from build123d import *

# Parameters (mm, degrees)
BOSS_EXTRUDE1_DEPTH     = 1.5
BOSS_EXTRUDE2_DEPTH     = 280
SKETCH4_W               = 410
SKETCH4_H               = 42.385541564
BOSS_EXTRUDE3_DEPTH     = 30
CUT_EXTRUDE1_DEPTH      = 616.233320702
CUT_EXTRUDE1_DEPTH_BACK = 616.233320702
SKETCH8_R               = 4.39
SKETCH8_R_2             = 2.39
BOSS_EXTRUDE5_DEPTH     = 15
SKETCH10_R              = 3
CUT_EXTRUDE2_DEPTH      = 1.5
SKETCH15_W              = 15
SKETCH15_H              = 1.5
SKETCH15_W_2            = 20
BOSS_EXTRUDE6_DEPTH     = 13
BOSS_EXTRUDE7_DEPTH     = 1.5
BOSS_EXTRUDE8_DEPTH     = 1.5
SKETCH20_R              = 2.415919743
SKETCH20_R_2            = 2
CUT_EXTRUDE5_DEPTH      = 1.5
SKETCH5_R               = 2
SKETCH5_R_2             = 10
CUT_EXTRUDE7_DEPTH      = 1.5
SKETCH21_W              = 300
SKETCH21_H              = 1.5
BOSS_EXTRUDE9_DEPTH     = 10
SKETCH22_W              = 300
SKETCH22_H              = 1.5
BOSS_EXTRUDE10_DEPTH    = 10
BOSS_EXTRUDE11_DEPTH    = 0.75
BOSS_EXTRUDE12_DEPTH    = 0.75
BOSS_EXTRUDE13_DEPTH    = 0.75
BOSS_EXTRUDE14_DEPTH    = 0.75
SKETCH27_W              = 200
SKETCH27_H              = 1.5
BOSS_EXTRUDE15_DEPTH    = 10
BOSS_EXTRUDE16_DEPTH    = 0.75
BOSS_EXTRUDE17_DEPTH    = 0.75
SKETCH30_R              = 24
SKETCH30_R_2            = 1.5
CUT_EXTRUDE8_DEPTH      = 1.5
SKETCH33_R              = 2
CUT_EXTRUDE9_DEPTH      = 1.5


with BuildPart() as part:
    # Sketch1 → Boss-Extrude1 (new body)
    with BuildSketch(Plane(origin=(0, 0, 0), x_dir=(1, 0, 0), z_dir=(0, 1, 0))):
        Polygon((-205, 237.826300096), (205, 237.826300096), (205, -292.173699904), (155, -292.173699904), (155, -362.173699904), (-205, -362.173699904), align=None)
    extrude(amount=BOSS_EXTRUDE1_DEPTH)

    # Sketch2 → Boss-Extrude2 (add)
    with BuildSketch(Plane(origin=(0, 1.5, 0), x_dir=(1, 0, 0), z_dir=(0, 1, 0))):
        Polygon((-205, 237.826300096), (-205, -362.173699904), (155, -362.173699904), (155, -292.173699904), (205, -292.173699904), (205, 237.826300096), align=None)
        Polygon((-203.5, 236.326300096), (-203.5, -360.673699904), (153.5, -360.673699904), (153.5, -290.673699904), (203.5, -290.673699904), (203.5, 236.326300096), align=None, mode=Mode.SUBTRACT)
    extrude(amount=BOSS_EXTRUDE2_DEPTH)

    # Sketch4 → Boss-Extrude3 (add)
    with BuildSketch(Plane(origin=(0, 0, -237.826300096), x_dir=(-1, 0, 0), z_dir=(0, 0, -1))):
        with Locations((0, 213.483316708)):
            Rectangle(SKETCH4_W, SKETCH4_H)
    extrude(amount=BOSS_EXTRUDE3_DEPTH)

    # Sketch3 → Cut-Extrude1 (cut, two sides: drawn at the far end of the back side and taken through both)
    with BuildSketch(Plane.ZY.offset(205).offset(-CUT_EXTRUDE1_DEPTH_BACK)):
        Polygon((362.173699904, 121.117558148), (228.195222706, 281.5), (362.173699904, 281.5), align=None)
    extrude(amount=CUT_EXTRUDE1_DEPTH + CUT_EXTRUDE1_DEPTH_BACK, mode=Mode.SUBTRACT)

    # Sketch8 → Boss-Extrude5 (add)
    # profile 1 of 2: a face of its own
    with BuildSketch(Plane(origin=(-203.5, 0, 0), x_dir=(0, 0, -1), z_dir=(1, 0, 0))):
        with Locations((-265.673699904, 172.2)):
            Circle(SKETCH8_R)
        with Locations((-265.673699904, 172.2)):
            Circle(SKETCH8_R_2, mode=Mode.SUBTRACT)
    # profile 2 of 2: a face of its own
    with BuildSketch(Plane(origin=(-203.5, 0, 0), x_dir=(0, 0, -1), z_dir=(1, 0, 0))):
        with Locations((-265.673699904, 16.5)):
            Circle(SKETCH8_R)
        with Locations((-265.673699904, 16.5)):
            Circle(SKETCH8_R_2, mode=Mode.SUBTRACT)
    extrude(amount=BOSS_EXTRUDE5_DEPTH)

    # Sketch10 → Cut-Extrude2 (cut)
    with BuildSketch(Plane.ZY.offset(-153.5)):
        with BuildLine():
            Line((334.423699904, 90.5), (320.423699904, 90.5))
            Line((320.423699904, 90.5), (320.423699904, 87.5))
            Line((320.423699904, 87.5), (316.173699904, 87.5))
            ThreePointArc((316.173699904, 87.5), (305.173699904, 76.5), (316.173699904, 65.5))
            Line((316.173699904, 65.5), (338.673699904, 65.5))
            ThreePointArc((338.673699904, 65.5), (349.673699904, 76.5), (338.673699904, 87.5))
            Line((338.673699904, 87.5), (334.423699904, 87.5))
            Line((334.423699904, 87.5), (334.423699904, 90.5))
        make_face()
        with Locations((301.473699904, 103.45)):
            Circle(SKETCH10_R)
        with Locations((353.373699904, 103.45)):
            Circle(SKETCH10_R)
        with Locations((301.473699904, 49.55)):
            Circle(SKETCH10_R)
        with Locations((353.373699904, 49.55)):
            Circle(SKETCH10_R)
    extrude(amount=-CUT_EXTRUDE2_DEPTH, mode=Mode.SUBTRACT)

    # Sketch15 → Boss-Extrude6 (add)
    with BuildSketch(Plane.ZY.offset(-203.5)):
        with Locations((-143.826300096, 251.386283415)):
            Rectangle(SKETCH15_W, SKETCH15_H)
        with Locations((136.673699904, 251.386283415)):
            Rectangle(SKETCH15_W_2, SKETCH15_H)
    extrude(amount=BOSS_EXTRUDE6_DEPTH)

    # Sketch17 → Boss-Extrude7 (add)
    with BuildSketch(Plane.XY.offset(-136.326300096)):
        Polygon((203.5, 250.636283415), (203.5, 235.636283415), (190.5, 250.636283415), align=None)
    extrude(amount=-BOSS_EXTRUDE7_DEPTH)

    # Sketch18 → Boss-Extrude8 (add)
    with BuildSketch(Plane.XY.offset(126.673699904)):
        Polygon((203.5, 250.636283415), (203.5, 235.636283415), (190.5, 250.636283415), align=None)
    extrude(amount=BOSS_EXTRUDE8_DEPTH)

    # Sketch20 → Cut-Extrude5 (cut)
    with BuildSketch(Plane(origin=(0, 252.136283415, 0), x_dir=(1, 0, 0), z_dir=(0, 1, 0))):
        with Locations(Location((198, 144.326300096, 0), (0, 0, 270))):
            Circle(SKETCH20_R)
        with Locations(Location((200.5, -139.673699904, 0), (0, 0, 270))):
            Circle(SKETCH20_R_2)
    extrude(amount=-CUT_EXTRUDE5_DEPTH, mode=Mode.SUBTRACT)

    # Sketch5 → Cut-Extrude7 (cut)
    with BuildSketch(Plane.ZY.offset(205)):
        with Locations((-116.326300096, 247.125857706)):
            Circle(SKETCH5_R)
        with Locations((-116.326300096, 223.125857706)):
            Circle(SKETCH5_R)
        with Locations((-92.326300096, 223.125857706)):
            Circle(SKETCH5_R)
        with Locations((-92.326300096, 247.125857706)):
            Circle(SKETCH5_R)
        with Locations((-104.326300096, 235.125857706)):
            Circle(SKETCH5_R_2)
        with Locations((-56.326300096, 247.125857706)):
            Circle(SKETCH5_R)
        with Locations((-56.326300096, 223.125857706)):
            Circle(SKETCH5_R)
        with Locations((-32.326300096, 223.125857706)):
            Circle(SKETCH5_R)
        with Locations((-32.326300096, 247.125857706)):
            Circle(SKETCH5_R)
        with Locations((-44.326300096, 235.125857706)):
            Circle(SKETCH5_R_2)
        with Locations((3.673699904, 247.125857706)):
            Circle(SKETCH5_R)
        with Locations((3.673699904, 223.125857706)):
            Circle(SKETCH5_R)
        with Locations((27.673699904, 223.125857706)):
            Circle(SKETCH5_R)
        with Locations((27.673699904, 247.125857706)):
            Circle(SKETCH5_R)
        with Locations((15.673699904, 235.125857706)):
            Circle(SKETCH5_R_2)
        with Locations((63.673699904, 247.125857706)):
            Circle(SKETCH5_R)
        with Locations((63.673699904, 223.125857706)):
            Circle(SKETCH5_R)
        with Locations((87.673699904, 223.125857706)):
            Circle(SKETCH5_R)
        with Locations((87.673699904, 247.125857706)):
            Circle(SKETCH5_R)
        with Locations((75.673699904, 235.125857706)):
            Circle(SKETCH5_R_2)
    extrude(amount=-CUT_EXTRUDE7_DEPTH, mode=Mode.SUBTRACT)

    # Sketch21 → Boss-Extrude9 (add)
    with BuildSketch(Plane(origin=(0, 0, -237.826300096), x_dir=(-1, 0, 0), z_dir=(0, 0, -1))):
        with Locations((0, 270.75)):
            Rectangle(SKETCH21_W, SKETCH21_H)
    extrude(amount=BOSS_EXTRUDE9_DEPTH)

    # Sketch22 → Boss-Extrude10 (add)
    with BuildSketch(Plane.ZY.offset(205)):
        with Locations((-7.826300096, 270.75)):
            Rectangle(SKETCH22_W, SKETCH22_H)
    boss_extrude10 = extrude(amount=BOSS_EXTRUDE10_DEPTH)

    # Sketch23 → Boss-Extrude11 (add, symmetric)
    with BuildSketch(Plane(origin=(0, 0, -77.826300096), x_dir=(-1, 0, 0), z_dir=(0, 0, -1))):
        Polygon((215, 270), (205, 270), (205, 260), align=None)
    boss_extrude11 = extrude(amount=BOSS_EXTRUDE11_DEPTH, both=True)

    # Sketch24 → Boss-Extrude12 (add, symmetric)
    with BuildSketch(Plane.XY.offset(52.173699904)):
        Polygon((-215, 270), (-205, 260), (-205, 270), align=None)
    boss_extrude12 = extrude(amount=BOSS_EXTRUDE12_DEPTH, both=True)

    # Sketch25 → Boss-Extrude13 (add, symmetric)
    with BuildSketch(Plane(origin=(100, 0, 0), x_dir=(0, 0, -1), z_dir=(1, 0, 0))):
        Polygon((247.826300096, 270), (237.826300096, 270), (237.826300096, 260), align=None)
    extrude(amount=BOSS_EXTRUDE13_DEPTH, both=True)

    # Sketch26 → Boss-Extrude14 (add, symmetric)
    with BuildSketch(Plane.ZY.offset(100)):
        Polygon((-247.826300096, 270), (-237.826300096, 260), (-237.826300096, 270), align=None)
    extrude(amount=BOSS_EXTRUDE14_DEPTH, both=True)

    # Mirror1: Boss-Extrude10, Boss-Extrude11, Boss-Extrude12 across plane
    add(boss_extrude10.mirror(Plane(origin=(0, 0, 0), x_dir=(0, 0, 1), z_dir=(1, 0, 0))))
    add(boss_extrude11.mirror(Plane(origin=(0, 0, 0), x_dir=(0, 0, 1), z_dir=(1, 0, 0))))
    add(boss_extrude12.mirror(Plane(origin=(0, 0, 0), x_dir=(0, 0, 1), z_dir=(1, 0, 0))))

    # Sketch27 → Boss-Extrude15 (add)
    with BuildSketch(Plane.XY.offset(362.173699904)):
        with Locations((-25, 110.367558148)):
            Rectangle(SKETCH27_W, SKETCH27_H)
    extrude(amount=BOSS_EXTRUDE15_DEPTH)

    # Sketch28 → Boss-Extrude16 (add, symmetric)
    with BuildSketch(Plane.ZY.offset(95)):
        Polygon((372.173699904, 109.617558148), (362.173699904, 109.617558148), (362.173699904, 99.617558148), align=None)
    extrude(amount=BOSS_EXTRUDE16_DEPTH, both=True)

    # Sketch29 → Boss-Extrude17 (add, symmetric)
    with BuildSketch(Plane(origin=(45, 0, 0), x_dir=(0, 0, -1), z_dir=(1, 0, 0))):
        Polygon((-372.173699904, 109.617558148), (-362.173699904, 99.617558148), (-362.173699904, 109.617558148), align=None)
    extrude(amount=BOSS_EXTRUDE17_DEPTH, both=True)

    # Sketch30 → Cut-Extrude8 (cut)
    with BuildSketch(Plane(origin=(205, 0, 0), x_dir=(0, 0, -1), z_dir=(1, 0, 0))):
        with Locations((-258.673699904, 160)):
            Circle(SKETCH30_R)
        with Locations((-284.673699904, 150)):
            Circle(SKETCH30_R_2)
        with Locations((-232.673699904, 150)):
            Circle(SKETCH30_R_2)
    extrude(amount=-CUT_EXTRUDE8_DEPTH, mode=Mode.SUBTRACT)

    # Sketch33 → Cut-Extrude9 (cut)
    with BuildSketch(Plane.ZY.offset(205)):
        with Locations((-180.626300096, 147.77)):
            Circle(SKETCH33_R)
        with Locations((-180.626300096, 28.39)):
            Circle(SKETCH33_R)
        with Locations((-8.926300096, 147.77)):
            Circle(SKETCH33_R)
        with Locations((-8.926300096, 28.39)):
            Circle(SKETCH33_R)
        with Locations((162.773699904, 147.77)):
            Circle(SKETCH33_R)
        with Locations((162.773699904, 28.39)):
            Circle(SKETCH33_R)
    extrude(amount=-CUT_EXTRUDE9_DEPTH, mode=Mode.SUBTRACT)


solid = part.part
Design review of the part built by this model. Coordinates are the model's own, in mm. A direction names the side the tool comes from. Coordinates: 2 decimals unless noted, no trailing zeros. Loops run counter-clockwise (first coordinate to the right, second up) from the corner with the lowest first, then second, coordinate; pieces in that order, holes last. Notation, with made-up numbers: (73, 86) -> (99, 86) arc R11 ccw to (99, 92) -> close; hole circle Ø10 at (30.25, 35.25). An arc over 180 degrees is marked (long way). Use a Markdown table: item, result. Add a question column.
Item 1: The part is to be moulded in two halves that separate along Y. For faces 1 (the cylindrical face through (-204.26, 225.364, 13.506)), 2 (the flat face through (3, 0, 58)), 3 (the flat face through (155, 101, 328)), 4 (the flat face through (199, 245, -137.826)), say which applies: +Y half, -Y half, draft (parallel to the pull), parting line (faces both ways), or undercut.
Item 2: We need section A-A, the plane x = 15. Write out the cut boundary in (y, z).
Item 3: We need section D-D, the plane y = 214.5. Write out the cut boundary in (x, z), and give its area (3 significant figures).
Item 4: Clearance check with flat-ended pins moving along their axes: P1, Ø5, axis at x = 117, z = -151.5, coming from the -Y side; P2, Ø23, axis at y = 235.13, z = 75.67, coming from the -X side; P3, Ø10, axis at x = -34.5, y = 85.5, coming from the -Z side; P4, Ø10.5, axis at x = 195.5, y = 241, coming from the +Z side. State where each tip first meets the part, or that it passes through.
Item 5: We need section B-B, the plane y = 76.5. Write out the cut boundary in (x, z).
Item 6: Machinability: for faces 5 (the flat face through (197, 252.136, 137)), 6 (the flat face through (3, 95, -237.826)), 7 (the cylindrical face through (204.26, 138.708, 247.599)), 8 (the flat face through (197, 250.636, 137)), which of the approach directions +Z, -Z, +X, -X, +Y, -Y give a long, thin tool a straight path to every point of the face, cutting with its end or side? Answer none if there is none.
Item 7: We need section C-C, the plane x = 85.5. Write out the cut boundary in (y, z).
Item 8: Wall thickness on L1, parallel to X at y = 74, z = -44.5; L2, parallel to Z at x = 63.5, y = 55.5; L3, parallel to Z at x = 183, y = 162.5: over which ranges is each line inside the solid? List them lowest first. Write a range as from..to.
Numbers:
| question | item | result |
|---|---|---|
| 1 | face 1 | undercut |
| 1 | face 2 | -Y half |
| 1 | face 3 | draft |
| 1 | face 4 | undercut |
| 2 | outline | (0, -237.83) -> (192.29, -237.83) -> (192.29, -267.83) -> (234.68, -267.83) -> (234.68, -237.83) -> (270, -237.83) -> (270, -247.83) -> (271.5, -247.83) -> (271.5, -237.83) -> (281.5, -237.83) -> (281.5, -236.33) -> (1.5, -236.33) -> (1.5, 360.67) -> (122.91, 360.67) -> (121.12, 362.17) -> (111.12, 362.17) -> (111.12, 372.17) -> (109.62, 372.17) -> (109.62, 362.17) -> (0, 362.17) -> close |
| 3 | outline | (-205, -267.83) -> (205, -267.83) -> (205, 284.16) -> (203.5, 284.16) -> (203.5, -236.33) -> (-203.5, -236.33) -> (-203.5, 284.16) -> (-205, 284.16) -> close |
| 3 | area | 14,500 mm^2 |
| 4 | P1 | stops at y = 0 |
| 4 | P2 | stops at x = -205 |
| 4 | P3 | stops at z = -237.83 |
| 4 | P4 | stops at z = 128.17 |
| 5 | outline | (-205, -237.83) -> (205, -237.83) -> (205, 292.17) -> (155, 292.17) -> (155, 305.17) -> (153.5, 305.17) -> (153.5, 290.67) -> (203.5, 290.67) -> (203.5, -236.33) -> (-203.5, -236.33) -> (-203.5, 360.67) -> (153.5, 360.67) -> (153.5, 349.67) -> (155, 349.67) -> (155, 362.17) -> (-205, 362.17) -> close |
| 6 | face 5 | +Z, +Y |
| 6 | face 6 | -Z, +X, -X, -Y |
| 6 | face 7 | +X |
| 6 | face 8 | +Z |
| 7 | outline | (0, -237.83) -> (192.29, -237.83) -> (192.29, -267.83) -> (234.68, -267.83) -> (234.68, -237.83) -> (270, -237.83) -> (270, -247.83) -> (271.5, -247.83) -> (271.5, -237.83) -> (281.5, -237.83) -> (281.5, -236.33) -> (1.5, -236.33) -> (1.5, 360.67) -> (122.91, 360.67) -> (121.12, 362.17) -> (0, 362.17) -> close |
| 8 | L1 | x = -205..-203.5, 203.5..205 |
| 8 | L2 | z = -237.83..-236.33, 360.67..362.17 |
| 8 | L3 | z = -237.83..-236.33, 290.67..292.17 |
